from build123d import *

# Parameters (mm, degrees)
EXTRUDE_1_DEPTH   = 20
EXTRUDE_1_2_DEPTH = 55


with BuildPart() as part:
    # 草图1 → Extrude 1 (new body)
    with BuildSketch(Plane(origin=(0, 0, 0), x_dir=(1, 0, 0), z_dir=(0, 1, 0))):
        with BuildLine():
            Line((0, 12.5), (100, 12.5))
            ThreePointArc((100, 12.5), (112.5, 0), (100, -12.5))
            Line((100, -12.5), (0, -12.5))
            ThreePointArc((0, -12.5), (-12.5, 0), (0, 12.5))
        make_face()
    extrude(amount=EXTRUDE_1_DEPTH)

    # 草图2 → Extrude 1 2 (add)
    with BuildSketch(Plane.XZ):
        with BuildLine():
            Line((100, 12.5), (0, 12.5))
            ThreePointArc((0, 12.5), (-12.5, 0), (0, -12.5))
            Line((0, -12.5), (100, -12.5))
            ThreePointArc((100, -12.5), (112.5, 0), (100, 12.5))
        make_face()
        with BuildLine():
            Line((100, 7.5), (0, 7.5))
            ThreePointArc((0, 7.5), (-7.5, 0), (0, -7.5))
            Line((0, -7.5), (100, -7.5))
            ThreePointArc((100, -7.5), (107.5, 0), (100, 7.5))
        make_face(mode=Mode.SUBTRACT)
    extrude(amount=-EXTRUDE_1_2_DEPTH)


solid = part.part
CAD build for the part. Positions are in the model's coordinates, mm. A direction names the side the tool comes from. Round coordinates to 2 decimals unless told otherwise and drop trailing zeros. Order: outer loops, then holes, each group sorted by start corner. A loop starts at its lowest first (then second) coordinate and runs counter-clockwise, first axis right, second up. Notation, with made-up numbers: (-37.75, 50) -> (-16.75, 50) arc R28 ccw to (-16.75, 70) -> close; hole circle Ø4 at (5, -11.5). An arc over 180 degrees is marked (long way). Write each question's results on one line, items separated by ' | '.
1. Cut at C-C (z = 0). Give the cut face in (x, y).
Findings below:
outline: (-12.5, 0) -> (112.5, 0) -> (112.5, 55) -> (107.5, 55) -> (107.5, 20) -> (-7.5, 20) -> (-7.5, 55) -> (-12.5, 55) -> close
2. Cut at A-A (y = 27). Give the cut face in (x, z), plus the area to 3 significant figures.
Findings below:
outline: (0, -12.5) -> (100, -12.5) arc R12.5 ccw to (100, 12.5) -> (0, 12.5) arc R12.5 ccw to start; hole (0, -7.5) -> (100, -7.5) arc R7.5 ccw to (100, 7.5) -> (0, 7.5) arc R7.5 ccw to start | area: 1,310 mm²
3. Cut at D-D (y = 11). Give the cut face in (x, z).
Findings below:
outline: (0, -12.5) -> (100, -12.5) arc R12.5 ccw to (100, 12.5) -> (0, 12.5) arc R12.5 ccw to start
4. Wall check: line 1 along Z through (x, y) = (94.5, 45.5); line 2 along Y through (x, z) = (9, 2.25); line 3 along X through (y, z) = (35.5, -4.5). Give the ranges that are in metal, low to high. Write a range as [from, to].
Findings below:
line 1: z = [-12.5, -7.5], [7.5, 12.5] | line 2: y = [0, 20] | line 3: x = [-11.66, -6], [106, 111.66]
5. 3-axis set-ups, long thin cutter, end or side, ignore diameter. For faces 4 (the face through (49, 37, -7.5)), 5 (the face through (49, 27, -12.5)): which of +Z, -Z, +X, -X, +Y, -Y reach the whole face in a straight line?
Findings below:
face 4: +Y | face 5: -Z, +X, -X, +Y, -Y
6. Cut at B-B (x = 79.5). Give the cut face in (y, z).
Findings below:
outline: (0, -12.5) -> (55, -12.5) -> (55, -7.5) -> (20, -7.5) -> (20, 7.5) -> (55, 7.5) -> (55, 12.5) -> (0, 12.5) -> close
7. Pull direction X, two halves, no side cores. Call faces 1 (the face through (51, 37, 7.5)), 2 (the face through (51, 27, 12.5)), 3 (the face through (112.497, 27.115, -0.275)): pulls with the +X half, pulls with the -X half, needs draft (parallel to the pull), parting line crosses it, or undercut.
Findings below:
face 1: undercut | face 2: needs draft | face 3: pulls with the +X half
8. Flat gauge pins, fed straight in: P1, Ø1, axis at y = 44.5, z = -2, coming from the +X side; P2, Ø3, axis at y = 12, z = 8, coming from the -X side; P3, Ø4, axis at y = 12.5, z = -6.5, coming from the +X side. Where does each tip first touch, or does it go through?
Findings below:
P1: stops at x = 112.41 | P2: stops at x = -10.68 | P3: stops at x = 111.66
